The listing builds one solid part. Answer for the finished solid, in the listing's coordinates (mm). Face numbers are marked on the shaded views. A direction names the side the tool comes from. Round coordinates to 2 decimals unless told otherwise and drop trailing zeros. Loops run counter-clockwise (first coordinate to the right, second up) from the corner with the lowest first, then second, coordinate; pieces in that order, holes last. Notation, with made-up numbers: (42.25, 27) -> (54.25, 27) arc R35 cw to (54.25, 59) -> close; hole circle Ø10 at (-30, -15). An arc over 180 degrees is marked (long way). Answer in a Markdown table with one row per item. Add a question column.
```python
from build123d import *

# Parameters (mm, degrees)
SKETCH_2_W          = 28
SKETCH_2_H          = 15
SKETCH_2_R          = 2.25
EXTRUDE_1_DEPTH     = 2
SKETCH_3_W          = 28
SKETCH_3_H          = 18
EXTRUDE_2_DEPTH     = 1.5
CHAMFER_1_SIZE      = 1.5
SKETCH_1_R          = 1.25
CUT_EXTRUDE_1_DEPTH = 109
FILLET_1_R          = 0.5
CHAMFER_2_SIZE      = 0.5


with BuildPart() as part:
    # 草图2 → 凸台-拉伸1 (new, symmetric)
    with BuildSketch(Plane.XY):
        Rectangle(SKETCH_2_W, SKETCH_2_H)
        with Locations((-10, 3.5)):
            Circle(SKETCH_2_R, mode=Mode.SUBTRACT)
        with Locations((10, 3.5)):
            Circle(SKETCH_2_R, mode=Mode.SUBTRACT)
    extrude(amount=EXTRUDE_1_DEPTH, both=True)

    # 草图3 → 凸台-拉伸2 (add, symmetric)
    with BuildSketch(Plane.XZ.offset(7.5)):
        Rectangle(SKETCH_3_W, SKETCH_3_H)
    extrude(amount=EXTRUDE_2_DEPTH, both=True)

    # 倒角1
    chamfer_1_edges = [part.edges().sort_by_distance(p)[0] for p in [
        (0, -6, 2),
        (0, -6, -2),
    ]]
    chamfer(chamfer_1_edges, length=CHAMFER_1_SIZE)

    # 草图1 → 切除-拉伸1 (cut)
    with BuildSketch(Plane(origin=(0, 0, 0), x_dir=(1, 0, 0), z_dir=(0, 1, 0))):
        with Locations(Location((-7, 5.5, 0), (0, 0, 270))):
            Circle(SKETCH_1_R)
        with Locations(Location((-7, -5.5, 0), (0, 0, 270))):
            Circle(SKETCH_1_R)
        with Locations(Location((7, -5.5, 0), (0, 0, 270))):
            Circle(SKETCH_1_R)
        with Locations(Location((7, 5.5, 0), (0, 0, 270))):
            Circle(SKETCH_1_R)
    extrude(amount=-CUT_EXTRUDE_1_DEPTH, mode=Mode.SUBTRACT)

    # 圆角1
    fillet_1_edges = [part.edges().sort_by_distance(p)[0] for p in [
        (-14, 1.5, 2),
        (14, -7.5, -9),
        (14, -6, -6.25),
        (-14, -6, 6.25),
        (-14, -7.5, 9),
        (0, -6, 9),
        (14, -7.5, 9),
        (0, -6, -9),
        (-14, -7.5, -9),
        (14, -9, 0),
        (0, -9, 9),
        (-14, -9, 0),
        (0, -9, -9),
        (-14, -6, -6.25),
        (0, -6, -3.5),
        (14, 1.5, -2),
        (0, -4.5, -2),
        (14, 1.5, 2),
        (0, -4.5, 2),
        (14, -6, 6.25),
        (0, -6, 3.5),
        (14, -5.25, -2.75),
        (-14, -5.25, -2.75),
        (14, -5.25, 2.75),
        (-14, -5.25, 2.75),
        (-14, 1.5, -2),
        (0, 7.5, -2),
        (-14, 7.5, 0),
        (14, 7.5, 0),
        (0, 7.5, 2),
    ]]
    fillet(fillet_1_edges, radius=FILLET_1_R)

    # 倒角2
    chamfer_2_edges = [part.edges().sort_by_distance(p)[0] for p in [
        (-12.25, 3.5, -2),
        (-12.25, 3.5, 2),
        (7.75, 3.5, -2),
        (7.75, 3.5, 2),
        (7, -9, -6.75),
        (7, -6, -6.75),
        (7, -6, 4.25),
        (7, -9, 4.25),
        (-7, -6, 4.25),
        (-7, -9, 4.25),
        (-7, -9, -6.75),
        (-7, -6, -6.75),
    ]]
    chamfer(chamfer_2_edges, length=CHAMFER_2_SIZE)


solid = part.part
```
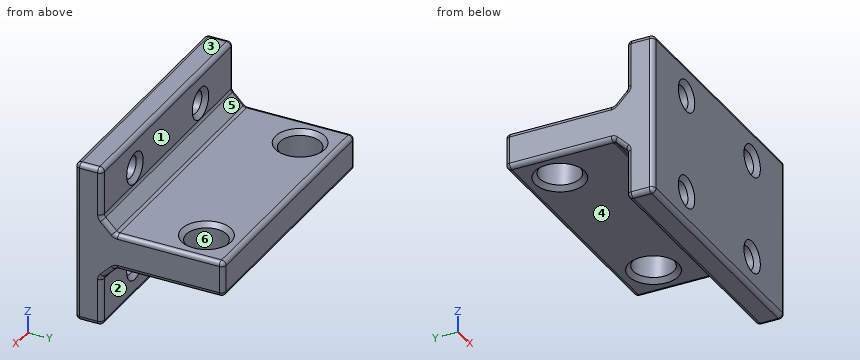
Item 1: Section D-D, the plane y = -2.25 is taken. Write down the section's boundary in (x, z).
Item 2: Section A-A, the plane x = -10 is taken. Write down the section's boundary in (y, z), and give its area (3 significant figures).
Item 3: Flat-ended cylindrical pins translate along their axes: P1, Ø5.5, axis at x = -5.5, z = 7, coming from the +Y side; P2, Ø7, axis at x = -10, y = 3.5, coming from the -Z side; P3, Ø4, axis at y = 2, z = 5.5, coming from the +X side; P4, Ø2, axis at x = -7, y = -1.5, coming from the +Z side. Find the tip coordinate at first contact, or state that the pin passes through.
Item 4: The mould has two halves that part along Y. Classify the marked faces 4, 5 and 6: +Y half, -Y half, draft (parallel to the pull), parting line (faces both ways), or undercut.
Item 5: Consider L1, parallel to X at y = -7.3, z = -5.5; L2, parallel to Y at x = 10, z = 0.9; L3, parallel to Z at x = -6.75, y = -2.25. Determine where each line is inside the solid, lowest interval first. Write a range as from..to.
Item 6: Section B-B, the plane z = -0.75 is taken. Write down the section's boundary in (x, y).
Item 7: Section C-C, the plane z = -5.5 is taken. Write down the section's boundary in (x, y), and give its area (3 significant figures).
Item 8: For the marked faces 1, 2 and 3, determine the directions among +Z, -Z, +X, -X, +Y, -Y from which every point of the face is accessible in a straight line to the end or side of a thin tool.
Here are the results:
| question | item | result |
|---|---|---|
| 1 | outline | (-14, -1.5) arc R0.5 ccw to (-13.5, -2) -> (13.5, -2) arc R0.5 ccw to (14, -1.5) -> (14, 1.5) arc R0.5 ccw to (13.5, 2) -> (-13.5, 2) arc R0.5 ccw to (-14, 1.5) -> close |
| 2 | outline | (-9, -8.5) arc R0.5 ccw to (-8.5, -9) -> (-6.5, -9) arc R0.5 ccw to (-6, -8.5) -> (-6, -3.71) arc R0.5 cw to (-5.85, -3.35) -> (-4.65, -2.15) arc R0.5 cw to (-4.29, -2) -> (0.75, -2) -> (1.25, -1.5) -> (1.25, 1.5) -> (0.75, 2) -> (-4.29, 2) arc R0.5 cw to (-4.65, 2.15) -> (-5.85, 3.35) arc R0.5 cw to (-6, 3.71) -> (-6, 8.5) arc R0.5 ccw to (-6.5, 9) -> (-8.5, 9) arc R0.5 ccw to (-9, 8.5) -> close; (5.75, -1.5) -> (6.25, -2) -> (7, -2) arc R0.5 ccw to (7.5, -1.5) -> (7.5, 1.5) arc R0.5 ccw to (7, 2) -> (6.25, 2) -> (5.75, 1.5) -> close |
| 2 | area | 91.4 mm² |
| 3 | P1 | stops at y = -6 |
| 3 | P2 | stops at z = -2 |
| 3 | P3 | passes through |
| 3 | P4 | stops at z = 2 |
| 4 | face 4 | draft |
| 4 | face 5 | +Y half |
| 4 | face 6 | undercut |
| 5 | L1 | x = -14..-8.25, -5.75..5.75, 8.25..14 |
| 5 | L2 | y = -9..1.25, 5.75..7.5 |
| 5 | L3 | z = -2..2 |
| 6 | outline | (-14, -8.5) arc R0.5 ccw to (-13.5, -9) -> (13.5, -9) arc R0.5 ccw to (14, -8.5) -> (14, 7) arc R0.5 ccw to (13.5, 7.5) -> (-13.5, 7.5) arc R0.5 ccw to (-14, 7) -> close; hole circle Ø4.5 at (-10, 3.5); hole circle Ø4.5 at (10, 3.5) |
| 7 | outline | (-14, -8.5) arc R0.5 ccw to (-13.5, -9) -> (-8.75, -9) -> (-8.25, -8.5) -> (-8.25, -6.5) -> (-8.75, -6) -> (-13.5, -6) arc R0.5 ccw to (-14, -6.5) -> close; (-5.75, -8.5) -> (-5.25, -9) -> (5.25, -9) -> (5.75, -8.5) -> (5.75, -6.5) -> (5.25, -6) -> (-5.25, -6) -> (-5.75, -6.5) -> close; (8.25, -8.5) -> (8.75, -9) -> (13.5, -9) arc R0.5 ccw to (14, -8.5) -> (14, -6.5) arc R0.5 ccw to (13.5, -6) -> (8.75, -6) -> (8.25, -6.5) -> close |
| 7 | area | 67.8 mm² |
| 8 | face 1 | +Z, +X, -X, +Y |
| 8 | face 2 | -Z, +X, -X, +Y |
| 8 | face 3 | +Z, +X, -X, +Y, -Y |
